Source: CAD feature listing. Evaluate the final solid. Frame: model axes, mm. A direction names the side the tool comes from. Round coordinates to 2 decimals unless told otherwise and drop trailing zeros. Write each loop counter-clockwise with the first axis right and the second up, starting at its lowest first coordinate (ties: lowest second). Pieces come first, ordered by that corner, then holes.
from build123d import *

# Parameters (mm, degrees)
SKETCH2_W           = 33
SKETCH2_H           = 18.5
BOSS_EXTRUDE1_DEPTH = 6
CUT_EXTRUDE1_DEPTH  = 1.25
SKETCH4_R           = 1.65
CUT_EXTRUDE2_DEPTH  = 20.844709622
CUT_EXTRUDE3_DEPTH  = 20.844709622


with BuildPart() as part:
    # Sketch2 → Boss-Extrude1 (new body)
    with BuildSketch(Plane(origin=(0, 0, 0), x_dir=(1, 0, 0), z_dir=(0, 1, 0))):
        Rectangle(SKETCH2_W, SKETCH2_H)
    extrude(amount=BOSS_EXTRUDE1_DEPTH)

    # Sketch3 → Cut-Extrude1 (cut)
    with BuildSketch(Plane(origin=(0, 6, 0), x_dir=(1, 0, 0), z_dir=(0, 1, 0))):
        with BuildLine():
            Line((-1, 9.25), (1, 9.25))
            Line((1, 9.25), (1, 5.8))
            Line((1, 5.8), (5.7, 5.8))
            ThreePointArc((5.7, 5.8), (8.528427125, 4.628427125), (9.7, 1.8))
            Line((9.7, 1.8), (9.7, -1.8))
            ThreePointArc((9.7, -1.8), (8.528427125, -4.628427125), (5.7, -5.8))
            Line((5.7, -5.8), (1, -5.8))
            Line((1, -5.8), (1, -9.25))
            Line((1, -9.25), (-1, -9.25))
            Line((-1, -9.25), (-1, -5.8))
            Line((-1, -5.8), (-5.7, -5.8))
            ThreePointArc((-5.7, -5.8), (-8.528427125, -4.628427125), (-9.7, -1.8))
            Line((-9.7, -1.8), (-9.7, 1.8))
            ThreePointArc((-9.7, 1.8), (-8.528427125, 4.628427125), (-5.7, 5.8))
            Line((-5.7, 5.8), (-1, 5.8))
            Line((-1, 5.8), (-1, 9.25))
        make_face()
        with BuildLine():
            Line((-5.7, -3.8), (5.7, -3.8))
            ThreePointArc((5.7, -3.8), (7.114213562, -3.214213562), (7.7, -1.8))
            Line((7.7, -1.8), (7.7, 1.8))
            ThreePointArc((7.7, 1.8), (7.114213562, 3.214213562), (5.7, 3.8))
            Line((5.7, 3.8), (-5.7, 3.8))
            ThreePointArc((-5.7, 3.8), (-7.114213562, 3.214213562), (-7.7, 1.8))
            Line((-7.7, 1.8), (-7.7, -1.8))
            ThreePointArc((-7.7, -1.8), (-7.114213562, -3.214213562), (-5.7, -3.8))
        make_face(mode=Mode.SUBTRACT)
    extrude(amount=-CUT_EXTRUDE1_DEPTH, mode=Mode.SUBTRACT)

    # Sketch4 → Cut-Extrude2 (cut, through all)
    with BuildSketch(Plane(origin=(0, 6, 0), x_dir=(1, 0, 0), z_dir=(0, 1, 0))):
        with Locations(Location((-12.5, 0, 0), (0, 0, 270))):
            Circle(SKETCH4_R)
        with Locations(Location((12.5, 0, 0), (0, 0, 270))):
            Circle(SKETCH4_R)
    extrude(amount=-CUT_EXTRUDE2_DEPTH, mode=Mode.SUBTRACT)

    # Sketch5 → Cut-Extrude3 (cut, through all)
    with BuildSketch(Plane(origin=(0, 6, 0), x_dir=(1, 0, 0), z_dir=(0, 1, 0))):
        with BuildLine():
            Line((-4.5, -1.5), (4.5, -1.5))
            ThreePointArc((4.5, -1.5), (6, 0), (4.5, 1.5))
            Line((4.5, 1.5), (-4.5, 1.5))
            ThreePointArc((-4.5, 1.5), (-6, 0), (-4.5, -1.5))
        make_face()
    extrude(amount=-CUT_EXTRUDE3_DEPTH, mode=Mode.SUBTRACT)


solid = part.part
1) Section query C-C on z = 0. Return the cut outline in (x, y), then the cut area to 3 significant figures.
Taken from the geometry:
outline: (-16.5, 0) - (-14.15, 0) - (-14.15, 6) - (-16.5, 6) - close; (-10.85, 0) - (-6, 0) - (-6, 6) - (-7.7, 6) - (-7.7, 4.75) - (-9.7, 4.75) - (-9.7, 6) - (-10.85, 6) - close; (6, 0) - (10.85, 0) - (10.85, 6) - (9.7, 6) - (9.7, 4.75) - (7.7, 4.75) - (7.7, 6) - (6, 6) - close; (14.15, 0) - (16.5, 0) - (16.5, 6) - (14.15, 6) - close
area: 81.4 mm2
2) Material intervals for line 1 (X direction, y = 1.75, z = 0); line 2 (Z direction, x = -0.5, y = 1.4); line 3 (Y direction, x = 5.5, z = 4), sorted ascending.
Taken from the geometry:
line 1: x = -16.5 to -14.15, -10.85 to -6, 6 to 10.85, 14.15 to 16.5
line 2: z = -9.25 to -1.5, 1.5 to 9.25
line 3: y = 0 to 4.75
3) Pull-direction query (Z, two-part tool) for faces 1 (the face through (0, 3, -9.25)), 2 (the face through (10, 6, 0)), 3 (the face through (-9.7, 5, 0)); classes: released by +Z, released by -Z, zero draft, split by the parting line, or undercut.
Taken from the geometry:
face 1: released by -Z
face 2: zero draft
face 3: undercut
4) Reachability of faces 4 (the face through (0, 3, -1.5)), 5 (the face through (-1, 5, -8)), 6 (the face through (-8.497, 5.384, 4.659)), 7 (the face through (-16.5, 3, 0)) from +Z, -Z, +X, -X, +Y, -Y: full face, straight path, thin tool, end or side. Return the list, or none.
Taken from the geometry:
face 4: +Y, -Y
face 5: -Z, +Y
face 6: +Y
face 7: +Z, -Z, -X, +Y, -Y
5) Section query D-D on y = 2. Return the cut outline in (x, z), then the cut area to 3 significant figures.
Taken from the geometry:
outline: (-16.5, -9.25) - (16.5, -9.25) - (16.5, 9.25) - (-16.5, 9.25) - close; hole circle Ø3.3 at (-12.5, 0); hole (-4.5, -1.5) - (4.5, -1.5) arc R1.5 ccw to (4.5, 1.5) - (-4.5, 1.5) arc R1.5 ccw to start; hole circle Ø3.3 at (12.5, 0)
area: 559 mm2
6) Section query A-A on y = 5.25. State how many separate pieces and enclosed holes the cut face has, then the cut area to 3 significant figures.
Taken from the geometry:
separate pieces: 3
enclosed holes: 3
area: 448 mm2
7) Section query B-B on x = 2.5. Return the cut outline in (y, z), then the cut area to 3 significant figures.
Taken from the geometry:
outline: (0, -9.25) - (6, -9.25) - (6, -5.8) - (4.75, -5.8) - (4.75, -3.8) - (6, -3.8) - (6, -1.5) - (0, -1.5) - close; (0, 1.5) - (6, 1.5) - (6, 3.8) - (4.75, 3.8) - (4.75, 5.8) - (6, 5.8) - (6, 9.25) - (0, 9.25) - close
area: 88.0 mm2
